from build123d import *

# Parameters (mm, degrees)
SKETCH_1_W                = 50.28
SKETCH_1_H                = 34.2
SKETCH_1_W_2              = 30.28
SKETCH_1_H_2              = 14.2
EXTRUDE_1_DEPTH           = 12.25
SKETCH_4_W                = 13
SKETCH_4_H                = 13.91
EXTRUDE_1_2_DEPTH         = 74.82
SKETCH_5_W                = 13.91
SKETCH_5_H                = 16.23
EXTRUDE_2_DEPTH           = 16
SKETCH_7_R                = 25.25
SKETCH_7_R_2              = 15.25
EXTRUDE_2_2_DEPTH         = 16.23
SKETCH_15_R               = 1.91
CUT_EXTRUDE_6_DEPTH       = 97.964478439
SKETCH_18_W               = 49.344544624
SKETCH_18_H               = 6.125
CUT_EXTRUDE_8_DEPTH       = 101.789238284
SKETCH_19_W               = 34.2
SKETCH_19_H               = 6.125
CUT_EXTRUDE_9_DEPTH       = 10
SKETCH_21_R               = 1.91
CUT_EXTRUDE_10_DEPTH      = 10
SKETCH_20_R               = 1.91
CUT_EXTRUDE_11_DEPTH      = 10
FILLET_START              = -7.1
FILLET_1_DEPTH            = 14.2
FILLET_2_DEPTH            = 14.2
SKETCH_29_W               = 13.91
SKETCH_29_H               = 74.82
EXTRUDE_5_DEPTH           = 10
SKETCH_30_W               = 10
SKETCH_30_H               = 58.59
CUT_EXTRUDE_13_DEPTH      = 97.964478439
SKETCH_32_W               = 34.2
SKETCH_32_H               = 5.745736365
EXTRUDE_6_DEPTH           = 10
CUT_EXTRUDE_16_DEPTH      = 50
CUT_EXTRUDE_16_DEPTH_BACK = 50
SKETCH_38_W               = 116.985630298
SKETCH_38_H               = 80.538350638
SKETCH_41_W               = 13.91
SKETCH_41_H               = 5.745736365
EXTRUDE_7_DEPTH           = 3
SKETCH_42_W               = 13
SKETCH_42_H               = 13.91
EXTRUDE_8_DEPTH           = 74.82
SKETCH_43_W               = 13.91
SKETCH_43_H               = 16.23
EXTRUDE_9_DEPTH           = 15.22
SKETCH_44_R               = 1.91
CUT_EXTRUDE_17_DEPTH      = 15.22
SKETCH_46_R               = 25.25
SKETCH_46_R_2             = 15.25
EXTRUDE_6_2_DEPTH         = 16.23
EXTRUDE_10_DEPTH          = 7.22
EXTRUDE_10_DEPTH_BACK     = 10
SKETCH_47_W               = 13.91
SKETCH_47_H               = 16.23
SKETCH_50_W               = 3.056753925
SKETCH_50_H               = 16.23
CUT_EXTRUDE_18_DEPTH      = 96.578211037
SKETCH_51_R               = 1.91
CUT_EXTRUDE_19_DEPTH      = 95.015226304
CUT_EXTRUDE_21_DEPTH      = 95.015226304
CUT_EXTRUDE_21_DEPTH_BACK = 95.015226304
SKETCH_54_W               = 96.956660426
SKETCH_54_H               = 45.351296872
CUT_EXTRUDE_22_DEPTH      = 60
SKETCH_59_W               = 19
SKETCH_59_H               = 37.38
EXTRUDE_12_DEPTH          = 10
SKETCH_60_R               = 4
CUT_EXTRUDE_25_DEPTH      = 24
SKETCH_61_W               = 19
SKETCH_61_H               = 10
EXTRUDE_13_DEPTH          = 26
SKETCH_62_R               = 4
CUT_EXTRUDE_26_DEPTH      = 24


with BuildPart() as part:
    # 草圖1 → Extrude 1 (new body)
    with BuildSketch(Plane(origin=(0, 0, 0), x_dir=(1, 0, 0), z_dir=(0, 1, 0))):
        Rectangle(SKETCH_1_W, SKETCH_1_H)
        Rectangle(SKETCH_1_W_2, SKETCH_1_H_2, mode=Mode.SUBTRACT)
    extrude(amount=EXTRUDE_1_DEPTH)

    # 草圖4 → Extrude 1 2 (add)
    with BuildSketch(Plane.XZ):
        with Locations((18.64, 0)):
            Rectangle(SKETCH_4_W, SKETCH_4_H)
    extrude(amount=EXTRUDE_1_2_DEPTH)

    # 草圖5 → Extrude 2 (add)
    with BuildSketch(Plane.ZY.offset(-12.14)):
        with Locations((0, -66.705)):
            Rectangle(SKETCH_5_W, SKETCH_5_H)
    extrude(amount=EXTRUDE_2_DEPTH)

    # 草圖7 → Extrude 2 2 (add)
    with BuildSketch(Plane(origin=(3.626674765, -74.82, 0), x_dir=(1, 0, 0), z_dir=(0, -1, 0))):
        with Locations((-30.978154344, 0)):
            Circle(SKETCH_7_R)
        with Locations((-30.978154344, 0)):
            Circle(SKETCH_7_R_2, mode=Mode.SUBTRACT)
    extrude(amount=-EXTRUDE_2_2_DEPTH)

    # 草圖15 → 除料-伸長6 (cut, through all)
    with BuildSketch(Plane(origin=(0, 0, -6.955), x_dir=(-1, 0, 0), z_dir=(0, 0, -1))):
        with Locations((-4.530883248, -66.705)):
            Circle(SKETCH_15_R)
    extrude(amount=-CUT_EXTRUDE_6_DEPTH, mode=Mode.SUBTRACT)

    # 草圖18 → 除料-伸長8 (cut, through all)
    with BuildSketch(Plane(origin=(0, 0, -17.1), x_dir=(-1, 0, 0), z_dir=(0, 0, -1))):
        with Locations((0.467727688, 9.1875)):
            Rectangle(SKETCH_18_W, SKETCH_18_H)
    extrude(amount=-CUT_EXTRUDE_8_DEPTH, mode=Mode.SUBTRACT)

    # 草圖19 → 除料-伸長9 (cut)
    with BuildSketch(Plane.ZY.offset(-24.204544624)):
        with Locations((0, 9.1875)):
            Rectangle(SKETCH_19_W, SKETCH_19_H)
    extrude(amount=-CUT_EXTRUDE_9_DEPTH, mode=Mode.SUBTRACT)

    # 草圖21 → 除料-伸長10 (cut)
    with BuildSketch(Plane(origin=(0, 6.125, 0), x_dir=(1, 0, 0), z_dir=(0, 1, 0))):
        with Locations(Location((17.69, 0, 0), (0, 0, 270))):
            Circle(SKETCH_21_R)
    extrude(amount=-CUT_EXTRUDE_10_DEPTH, mode=Mode.SUBTRACT)

    # 草圖20 → 除料-伸長11 (cut)
    with BuildSketch(Plane(origin=(0, 6.125, 0), x_dir=(1, 0, 0), z_dir=(0, 1, 0))):
        with Locations(Location((-17.395, 0, 0), (0, 0, 270))):
            Circle(SKETCH_20_R)
    extrude(amount=-CUT_EXTRUDE_11_DEPTH, mode=Mode.SUBTRACT)

    # 圓角1: read off the stored shape, not the designer's step
    # 圓角1 outline → 圓角1 (cut)
    with BuildSketch(Plane.XY.offset(FILLET_START)):
        with BuildLine():
            add(Edge.make_bspline(
                [(-15.14, 0), (-21.974170252, 5.199829476), (-25.14, 5.745736365)],
                knots=[0, 0, 0, 0.664102345, 0.664102345, 0.664102345], degree=2, weights=[1, 2.223777218, 1.822127795]))
            Line((-15.14, 0), (-15.14, 6.125))
            Line((-15.14, 6.125), (-25.14, 6.125))
            Line((-25.14, 6.125), (-25.14, 5.745736365))
        make_face()
    extrude(amount=FILLET_1_DEPTH, mode=Mode.SUBTRACT)

    # 圓角2: read off the stored shape, not the designer's step
    # 圓角2 outline → 圓角2 (cut)
    with BuildSketch(Plane.XY.offset(FILLET_START)):
        with BuildLine():
            Line((15.14, 6.125), (15.14, 0))
            add(Edge.make_bspline(
                [(15.14, 0), (21.974170252, 5.199829476), (25.14, 5.745736365)],
                knots=[0, 0, 0, 0.664102345, 0.664102345, 0.664102345], degree=2, weights=[1, 2.223777218, 1.822127795]))
            Line((25.14, 5.745736365), (25.14, 6.125))
            Line((25.14, 6.125), (15.14, 6.125))
        make_face()
    extrude(amount=FILLET_2_DEPTH, mode=Mode.SUBTRACT)

    # 草圖29 → 填料-伸長5 (add)
    with BuildSketch(Plane(origin=(25.14, 0, 0), x_dir=(0, 0, -1), z_dir=(1, 0, 0))):
        with Locations((0, -37.41)):
            Rectangle(SKETCH_29_W, SKETCH_29_H)
    extrude(amount=EXTRUDE_5_DEPTH)

    # 草圖30 → 除料-伸長13 (cut, through all)
    with BuildSketch(Plane.XY.offset(6.955)):
        with Locations((17.14, -29.295)):
            Rectangle(SKETCH_30_W, SKETCH_30_H)
    extrude(amount=-CUT_EXTRUDE_13_DEPTH, mode=Mode.SUBTRACT)

    # 草圖32 → Extrude 6 (add)
    with BuildSketch(Plane(origin=(25.14, 0, 0), x_dir=(0, 0, -1), z_dir=(1, 0, 0))):
        with Locations((0, 2.872868182)):
            Rectangle(SKETCH_32_W, SKETCH_32_H)
    extrude(amount=EXTRUDE_6_DEPTH)

    # 草圖38 → 除料-伸長16 (cut, two sides: drawn at the far end of the back side and taken through both)
    with BuildSketch(Plane(origin=(0, 0, -6.955), x_dir=(-1, 0, 0), z_dir=(0, 0, -1)).offset(-CUT_EXTRUDE_16_DEPTH_BACK)):
        with Locations((7.268869252, -40.269175319)):
            Rectangle(SKETCH_38_W, SKETCH_38_H)
    extrude(amount=CUT_EXTRUDE_16_DEPTH + CUT_EXTRUDE_16_DEPTH_BACK, mode=Mode.SUBTRACT)

    # 草圖41 → 填料-伸長7 (add)
    with BuildSketch(Plane(origin=(35.14, 0, 0), x_dir=(0, 0, -1), z_dir=(1, 0, 0))):
        with Locations((0, 2.872868182)):
            Rectangle(SKETCH_41_W, SKETCH_41_H)
    extrude(amount=EXTRUDE_7_DEPTH)

    # 草圖42 → 填料-伸長8 (add)
    with BuildSketch(Plane(origin=(0, 0, 0), x_dir=(-1, 0, 0), z_dir=(0, -1, 0))):
        with Locations((-31.64, 0)):
            Rectangle(SKETCH_42_W, SKETCH_42_H)
    extrude(amount=EXTRUDE_8_DEPTH)

    # 草圖43 → 填料-伸長9 (add)
    with BuildSketch(Plane.ZY.offset(-25.14)):
        with Locations((0, -66.705)):
            Rectangle(SKETCH_43_W, SKETCH_43_H)
    extrude(amount=EXTRUDE_9_DEPTH)

    # 草圖44 → 除料-伸長17 (cut)
    with BuildSketch(Plane(origin=(0, 0, -6.955), x_dir=(-1, 0, 0), z_dir=(0, 0, -1))):
        with Locations(Location((-17.524895264, -66.705, 0), (0, 0, 90))):
            Circle(SKETCH_44_R)
    extrude(amount=-CUT_EXTRUDE_17_DEPTH, mode=Mode.SUBTRACT)

    # 草圖46 → Extrude 6 2 (add)
    with BuildSketch(Plane(origin=(0, -58.59, 0), x_dir=(1, 0, 0), z_dir=(0, 1, 0))):
        with Locations((-14.35, 0)):
            Circle(SKETCH_46_R)
        with Locations((-14.35, 0)):
            Circle(SKETCH_46_R_2, mode=Mode.SUBTRACT)
    extrude(amount=-EXTRUDE_6_2_DEPTH)

    # 草圖47 → 填料-伸長10 (add, two sides: drawn at the far end of the back side and taken through both)
    with BuildSketch(Plane(origin=(-40, 0, 0), x_dir=(0, 0, -1), z_dir=(1, 0, 0)).offset(-EXTRUDE_10_DEPTH_BACK)):
        with Locations((0, -66.705)):
            Rectangle(SKETCH_47_W, SKETCH_47_H)
    extrude(amount=EXTRUDE_10_DEPTH + EXTRUDE_10_DEPTH_BACK)

    # 草圖50 → 除料-伸長18 (cut, through all)
    with BuildSketch(Plane(origin=(0, 0, -6.955), x_dir=(-1, 0, 0), z_dir=(0, 0, -1))):
        with Locations((48.471623038, -66.705)):
            Rectangle(SKETCH_50_W, SKETCH_50_H)
    extrude(amount=-CUT_EXTRUDE_18_DEPTH, mode=Mode.SUBTRACT)

    # 草圖51 → 除料-伸長19 (cut, through all)
    with BuildSketch(Plane(origin=(0, 0, -6.955), x_dir=(-1, 0, 0), z_dir=(0, 0, -1))):
        with Locations((42.786508152, -66.705)):
            Circle(SKETCH_51_R)
    extrude(amount=-CUT_EXTRUDE_19_DEPTH, mode=Mode.SUBTRACT)

    # 草圖53 → 除料-伸長21 (cut, two sides: drawn at the far end of the back side and taken through both)
    with BuildSketch(Plane.XY.offset(6.955).offset(-CUT_EXTRUDE_21_DEPTH_BACK)):
        Polygon((25.14, -58.59), (25.14, -81.637244924), (42.795360098, -81.637244924), (56.21630317, 11.638309425), (-41.644740061, 8.95412081), (-39.519757408, -16.545671026), (25.14, -20.795636332), align=None)
    extrude(amount=CUT_EXTRUDE_21_DEPTH + CUT_EXTRUDE_21_DEPTH_BACK, mode=Mode.SUBTRACT)

    # 草圖54 → 除料-伸長22 (cut)
    with BuildSketch(Plane(origin=(0, -58.59, 0), x_dir=(1, 0, 0), z_dir=(0, 1, 0))):
        with Locations((-23.338330213, -22.675648436)):
            Rectangle(SKETCH_54_W, SKETCH_54_H)
    extrude(amount=-CUT_EXTRUDE_22_DEPTH, mode=Mode.SUBTRACT)

    # 草圖59 → 填料-伸長12 (add)
    with BuildSketch(Plane.XY.offset(-30)):
        with Locations((-14.576753925, -48.015)):
            Rectangle(SKETCH_59_W, SKETCH_59_H)
    extrude(amount=EXTRUDE_12_DEPTH)

    # 草圖60 → 除料-伸長25 (cut)
    with BuildSketch(Plane(origin=(0, -29.325, 0), x_dir=(1, 0, 0), z_dir=(0, 1, 0))):
        with Locations((-14.576753925, 20)):
            Circle(SKETCH_60_R)
    extrude(amount=-CUT_EXTRUDE_25_DEPTH, mode=Mode.SUBTRACT)

    # 草圖61 → 填料-伸長13 (add)
    with BuildSketch(Plane(origin=(0, -29.325, 0), x_dir=(1, 0, 0), z_dir=(0, 1, 0))):
        with Locations((-14.576753925, 25)):
            Rectangle(SKETCH_61_W, SKETCH_61_H)
    extrude(amount=EXTRUDE_13_DEPTH)

    # 草圖62 → 除料-伸長26 (cut)
    with BuildSketch(Plane(origin=(0, -3.325, 0), x_dir=(1, 0, 0), z_dir=(0, 1, 0))):
        with Locations((-14.576753925, 20)):
            Circle(SKETCH_62_R)
    extrude(amount=-CUT_EXTRUDE_26_DEPTH, mode=Mode.SUBTRACT)


solid = part.part
Geometry: final body of the model. Coordinates: model frame, mm. A direction names the side the tool comes from. Give positions to 0.01 mm unless a question says otherwise; leave off trailing zeros. Loops run counter-clockwise (first coordinate to the right, second up) from the corner with the lowest first, then second, coordinate; pieces in that order, holes last. Notation, with made-up numbers: (-9, -28) - (40, -28) arc R9 cw to (40, -21) - close; hole circle Ø2 at (-28.75, 4). An arc over 180 degrees is marked (long way). Answer as CSV lines item,"result". Start each with the question number.
1. Section C-C, the plane z = -13. Return loops of the section in (x, y).
2. Section B-B, the plane y = -52. Return loops of the section in (x, z).
3. Reachability of faces 4 (the face through (-19, -31, -20)), 5 (the face through (-15, -27.325, -22)), 6 (the face through (-43, -69, -6.955)), 7 (the face through (-14.5, -41.2, -24)), 8 (the face through (-38, -67, 0)) from +Z, -Z, +X, -X, +Y, -Y: full face, straight path, thin tool, end or side. Return the list, or none.
4. Section A-A, the plane z = -4.5. Return loops of the section in (x, y) (1 decimal).
5. Pin query (flat end, axial travel): P1, Ø5, axis at y = -30.5, z = -24.5, coming from the -X side; P2, Ø7.5, axis at x = -16, z = -25.5, coming from the -Y side; P3, Ø15, axis at x = -15, y = -39, coming from the +Z side; P4, Ø3, axis at y = -34, z = -20, coming from the +X side. Return the tip coordinate at first contact, or that it passes through.
6. Section D-D, the plane x = -14.35. Return loops of the section in (y, z) (3 decimals), plus the area to 3 significant figures.
7. Draft query along X for faces 1 (the face through (-11, -58.59, -17)), 2 (the face through (25.14, -67, -4)), 3 (the face through (-14.5, -15.2, -24)). Return one class per face: released by +X, released by -X, zero draft, split by the parting line, or undercut.
8. Ray query, L1, parallel to X at y = -18, z = -21.5; L2, parallel to Z at x = -39.5, y = -59 (3 decimals); L3, parallel to Z at x = -7, y = -33.5. Return the intervals inside material, ascending.
Answers:
1,outline,"(-36, -74.82) - (-22.32, -74.82) - (-22.32, -58.59) - (-36, -58.59) - close; (-6.38, -74.82) - (7.3, -74.82) - (7.3, -58.59) - (-6.38, -58.59) - close"
2,outline,"(-24.08, -30) - (-5.08, -30) - (-5.08, -20) - (-10.58, -20) arc R4 cw to (-18.58, -20) - (-24.08, -20) - close"
3,face 4,"+Z, +X, -X, +Y"
3,face 5,"+Z, +Y"
3,face 6,"-Z, -X, +Y, -Y"
3,face 7,"+Z"
3,face 8,"+Z, +X, -X, +Y, -Y"
4,outline,"(-46.9, -74.8) - (-28.9, -74.8) - (-28.9, -58.6) - (-46.9, -58.6) - close; (0.2, -74.8) - (25.1, -74.8) - (25.1, -58.6) - (0.2, -58.6) - close; hole circle Ø3.8 at (-42.8, -66.7); hole circle Ø3.8 at (17.5, -66.7)"
5,P1,"stops at x = -24.08"
5,P2,"stops at y = -74.82"
5,P3,"stops at z = -20"
5,P4,"stops at x = -5.08"
6,outline,"(-74.82, -25.25) - (-66.705, -25.25) - (-66.705, -30) - (-3.325, -30) - (-3.325, -23.994) - (-27.325, -23.994) - (-27.325, -20) - (-29.325, -20) - (-29.325, -23.994) - (-53.325, -23.994) - (-53.325, -20) - (-58.59, -20) - (-58.59, -15.25) - (-74.82, -15.25) - close"
6,area,"562 mm2"
7,face 1,"zero draft"
7,face 2,"released by +X"
7,face 3,"undercut"
8,L1,"x = -24.08 to -18.28, -10.87 to -5.08"
8,L2,"z = -6.955 to 0"
8,L3,"z = -30 to -20"
